Build history of the part. All positions in model axes, mm. A direction names the side the tool comes from. Round coordinates to 2 decimals unless told otherwise and drop trailing zeros. Write each loop counter-clockwise with the first axis right and the second up, starting at its lowest first coordinate (ties: lowest second). Pieces come first, ordered by that corner, then holes. Notation, with made-up numbers: (-29.5, 77.5) -> (19.5, 77.5) arc R14 ccw to (19.5, 87.5) -> close; hole circle Ø11 at (88.5, 61). An arc over 180 degrees is marked (long way). One line per question, with ' | ' between items.
from build123d import *

# Parameters (mm, degrees)
BOSS_EXTRUDE1_DEPTH     = 199.23125
CUT_EXTRUDE3_DEPTH      = 223.035867827
CUT_EXTRUDE3_DEPTH_BACK = 223.035867827
SKETCH4_R               = 5.588
SKETCH5_W               = 44.45
SKETCH5_H               = 111.125148887
BOSS_EXTRUDE3_DEPTH     = 3.175


with BuildPart() as part:
    # Sketch1 → Boss-Extrude1 (new, symmetric)
    with BuildSketch(Plane.XY):
        Polygon((3.175, 88.9), (3.175, 3.175), (44.45, 3.175), (44.45, 0), (0, 0), (0, 88.9), align=None)
    extrude(amount=BOSS_EXTRUDE1_DEPTH, both=True)

    # Sketch4 → Cut-Extrude3 (cut, two sides: drawn at the far end of the back side and taken through both)
    with BuildSketch(Plane(origin=(3.175, 0, 0), x_dir=(0, 0, -1), z_dir=(1, 0, 0)).offset(-CUT_EXTRUDE3_DEPTH_BACK)):
        with Locations(Location((148.43125, 44.45, 0), (0, 0, 270))):
            Circle(SKETCH4_R)
        Polygon((-199.23125, 88.9), (-132.556001855, 0), (-199.23125, 0), align=None)
    extrude(amount=CUT_EXTRUDE3_DEPTH + CUT_EXTRUDE3_DEPTH_BACK, mode=Mode.SUBTRACT)

    # Sketch5 → Boss-Extrude3 (add)
    with BuildSketch(Plane(origin=(0, -63.626947194, 84.835613859), x_dir=(1, 0, 0), z_dir=(0, -0.6000014291326674, 0.7999989281485049))):
        with Locations((22.225, 135.096364997)):
            Rectangle(SKETCH5_W, SKETCH5_H)
    extrude(amount=BOSS_EXTRUDE3_DEPTH)


solid = part.part
(1) 3-axis set-ups, long thin cutter, end or side, ignore diameter. For faces 1 (the flat face through (23.524, 46.638, 167.534)), 2 (the flat face through (0, 36, -9)): which of +Z, -Z, +X, -X, +Y, -Y reach the whole face in a straight line?
Calculated:
face 1: -Z, +X, +Y | face 2: +Z, -Z, -X, +Y, -Y
(2) Slice it at A-A (x = 12). Write the cut outline in (y, z) (3 decimals), then the cut area to 3 significant figures.
Calculated:
outline: (-1.905, 135.096) -> (0, 132.556) -> (0, -199.231) -> (3.175, -199.231) -> (3.175, 134.937) -> (88.9, 199.231) -> (86.995, 201.771) -> close | area: 1,410 mm2
(3) Slice it at D-D (y = 63). Write the cut outline in (x, z) (3 decimals).
Calculated:
outline: (0, -199.231) -> (3.175, -199.231) -> (3.175, 179.806) -> (44.45, 179.806) -> (44.45, 183.775) -> (0, 183.775) -> close
(4) Slice it at C-C (z = -1). Write the cut outline in (x, y) (3 decimals), then the cut area to 3 significant figures.
Calculated:
outline: (0, 0) -> (44.45, 0) -> (44.45, 3.175) -> (3.175, 3.175) -> (3.175, 88.9) -> (0, 88.9) -> close | area: 413 mm2
(5) Wall check: line 1 (X direction, y = 76.5, z = 179.5) (3 decimals); line 2 (Y direction, x = 2.5, z = 127.5). Give the ranges that are in metal, low to high. Write a range as from..to.
Calculated:
line 1: 0..3.175 | line 2: 0..88.9
(6) Mould opens along Y. For faces 3 (the flat face through (23, 0, -31)), 4 (the cylindrical face through (1.57, 45.18, -153.97)), 5 (the flat face through (3, 31, -199.231)), 6 (the flat face through (24, 3.175, -30)) say: pulls with the +Y half, pulls with the -Y half, needs draft (parallel to the pull), parting line crosses it, or undercut.
Calculated:
face 3: pulls with the -Y half | face 4: undercut | face 5: needs draft | face 6: pulls with the +Y half
(7) Drop flat-ended pins along their axis: pin 1 (5 mm diameter, centred on x = 9, z = 103, fed in from -Y); pin 2 (1 mm diameter, centred on y = 15.5, z = 150.5, fed in from -X); pin 3 (2 mm diameter, centred on x = 10, y = 22, fed in from +Z); pin 4 (2 mm diameter, centred on x = 33.5, y = 8, fed in from +Z). Give the stop position or say it passes through.
Calculated:
pin 1: y = 0 | pin 2: through | pin 3: z = 153.77 | pin 4: z = 143.27
(8) Slice it at B-B (y = 44.45). Write the cut outline in (x, z) (3 decimals), then the cut area to 3 significant figures.
Calculated:
outline: (0, -199.231) -> (3.175, -199.231) -> (3.175, -154.019) -> (0, -154.019) -> close; (0, -142.843) -> (3.175, -142.843) -> (3.175, 165.894) -> (44.45, 165.894) -> (44.45, 169.862) -> (0, 169.862) -> close | area: 1,300 mm2
